```python
from build123d import *

# Parameters (mm, degrees)
BOSS_EXTRUDE1_DEPTH = 126
SKETCH2_R           = 1.5
CUT_EXTRUDE1_DEPTH  = 45
SKETCH3_R           = 1.5
CUT_EXTRUDE3_DEPTH  = 55
CUT_EXTRUDE6_DEPTH  = 45


with BuildPart() as part:
    # Sketch1 → Boss-Extrude1 (new body)
    with BuildSketch(Plane(origin=(0, 0, 0), x_dir=(0, 0, -1), z_dir=(1, 0, 0))):
        Polygon((-95, -3.570472346), (-95, 46.429527654), (-44, 46.429527654), (-44, 51.429527654), (-95, 51.429527654), (-95, 91.429527654), (-25, 91.429527654), (-25, 96.429527654), (-90, 96.429527654), (-100, 96.429527654), (-100, 86.429527654), (-100, -8.570472346), (-90, -8.570472346), (-15, -8.570472346), (-15, -3.570472346), align=None)
    boss_extrude1 = extrude(amount=BOSS_EXTRUDE1_DEPTH)

    # Sketch2 → Cut-Extrude1 (cut)
    with BuildSketch(Plane(origin=(0, 96.429527654, 0), x_dir=(1, 0, 0), z_dir=(0, 1, 0))):
        with Locations(Location((3, -28, 0), (0, 0, 270))):
            Circle(SKETCH2_R)
        with Locations(Location((123, -28, 0), (0, 0, 270))):
            Circle(SKETCH2_R)
    cut_extrude1 = extrude(amount=-CUT_EXTRUDE1_DEPTH, mode=Mode.SUBTRACT)

    # Sketch3 → Cut-Extrude3 (cut)
    with BuildSketch(Plane(origin=(0, 51.429527654, 0), x_dir=(1, 0, 0), z_dir=(0, 1, 0))):
        with Locations(Location((3, -47, 0), (0, 0, 270))):
            Circle(SKETCH3_R)
        with Locations(Location((123, -47, 0), (0, 0, 270))):
            Circle(SKETCH3_R)
        with BuildLine():
            Line((6, -74), (6, -44))
            Line((6, -44), (120, -44))
            Line((120, -44), (120, -74))
            ThreePointArc((120, -74), (117.071067812, -81.071067812), (110, -84))
            Line((110, -84), (16, -84))
            ThreePointArc((16, -84), (8.928932188, -81.071067812), (6, -74))
        make_face()
    cut_extrude3 = extrude(amount=-CUT_EXTRUDE3_DEPTH, mode=Mode.SUBTRACT)

    # Mirror2: Boss-Extrude1, Cut-Extrude1, Cut-Extrude3 across plane
    add(boss_extrude1.mirror(Plane(origin=(0, 0, 15), x_dir=(1, 0, 0), z_dir=(0, 0, -1))))
    add(cut_extrude1.mirror(Plane(origin=(0, 0, 15), x_dir=(1, 0, 0), z_dir=(0, 0, -1))), mode=Mode.SUBTRACT)
    add(cut_extrude3.mirror(Plane(origin=(0, 0, 15), x_dir=(1, 0, 0), z_dir=(0, 0, -1))), mode=Mode.SUBTRACT)

    # Sketch4 → Cut-Extrude6 (cut)
    with BuildSketch(Plane(origin=(0, 96.429527654, 0), x_dir=(1, 0, 0), z_dir=(0, 1, 0))):
        with BuildLine():
            Line((9, -25), (9, -80))
            ThreePointArc((9, -80), (11.928932188, -87.071067812), (19, -90))
            Line((19, -90), (107, -90))
            ThreePointArc((107, -90), (114.071067812, -87.071067812), (117, -80))
            Line((117, -80), (117, -25))
            Line((117, -25), (9, -25))
        make_face()
    cut_extrude6 = extrude(amount=-CUT_EXTRUDE6_DEPTH, mode=Mode.SUBTRACT)

    # Mirror5: Cut-Extrude6 across plane
    add(cut_extrude6.mirror(Plane(origin=(0, 0, 15), x_dir=(1, 0, 0), z_dir=(0, 0, -1))), mode=Mode.SUBTRACT)


solid = part.part
```
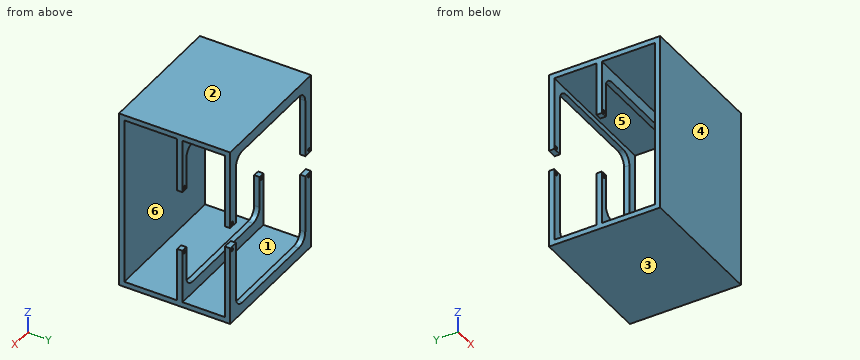
Design review of the part built by this model. Coordinates are the model's own, in mm. Face numbers are marked on the shaded views. A direction names the side the tool comes from. Give positions to 0.01 mm unless a question says otherwise; leave off trailing zeros. Order: outer loops, then holes, each group sorted by start corner. A loop starts at its lowest first (then second) coordinate and runs counter-clockwise, first axis right, second up. Notation, with made-up numbers: (75, 52) -> (84, 52) arc R21 cw to (84, 86) -> close; hole circle Ø2 at (10, 3). An arc over 180 degrees is marked (long way). Write item = value, one per line. Start each with the question number.
(1) We need section C-C on z = -8.5. Write out the cut boundary in (x, y).
(2) Mouldability with a two-part tool opening along Z and no side actions: class the marked faces 3, 4, 5 and 6 as +Z half, -Z half, draft (parallel to the pull), parting line (faces both ways), or undercut.
(3) We need section A-A on z = 60.5. Write out the cut boundary in (x, y).
(4) For pin 1 (3 mm diameter, centred on x = 72, z = -0.5, fed in from +Y), flat-tipped, find the tip position at first contact; note if it passes through.
(5) We need section B-B on y = 34.5. Write out the cut boundary in (x, z).
(6) We need section D-D on x = 42.5. Write out the cut boundary in (y, z), plus the area to 3 significant figures.
(7) For the marked faces 1 and 2, list the 3-axis set-ups (+Z, -Z, +X, -X, +Y, -Y) from which the entire face can be reached by the end or side of a thin tool; tool diameter is ignored.
(8) To check wall thickness, follow line 1 along X through (y, z) = (94.9, 2); line 2 along X through (y, z) = (48, 47); line 3 along Z through (x, y) = (123, 49.1). State the ranges of each line that lie inside material, in increasing order.
Numbers:
q1.outline = (0, -8.57) -> (126, -8.57) -> (126, -3.57) -> (0, -3.57) -> close; (0, 91.43) -> (9, 91.43) -> (9, 96.43) -> (0, 96.43) -> close; (117, 91.43) -> (126, 91.43) -> (126, 96.43) -> (117, 96.43) -> close
q2.face_3 = -Z half
q2.face_4 = draft
q2.face_5 = undercut
q2.face_6 = undercut
q3.outline = (0, -8.57) -> (126, -8.57) -> (126, -3.57) -> (0, -3.57) -> close; (0, 46.43) -> (6, 46.43) -> (6, 51.43) -> (0, 51.43) -> close; (0, 91.43) -> (9, 91.43) -> (9, 96.43) -> (0, 96.43) -> close; (117, 91.43) -> (126, 91.43) -> (126, 96.43) -> (117, 96.43) -> close; (120, 46.43) -> (126, 46.43) -> (126, 51.43) -> (120, 51.43) -> close
q4.pin_1 = -3.57
q5.outline = (0, -70) -> (126, -70) -> (126, -65) -> (0, -65) -> close; (0, 95) -> (126, 95) -> (126, 100) -> (0, 100) -> close
q6.outline = (-8.57, -70) -> (96.43, -70) -> (96.43, -60) -> (91.43, -60) -> (91.43, -65) -> (51.43, -65) -> (51.43, -54) -> (46.43, -54) -> (46.43, -65) -> (-3.57, -65) -> (-3.57, 95) -> (46.43, 95) -> (46.43, 84) -> (51.43, 84) -> (51.43, 95) -> (91.43, 95) -> (91.43, 90) -> (96.43, 90) -> (96.43, 100) -> (-8.57, 100) -> close
q6.area = 2,010 mm^2
q7.face_1 = +X, -X
q7.face_2 = +Z, +X, -X, +Y, -Y
q8.line_1 = 0 to 1.5, 4.5 to 9, 117 to 121.5, 124.5 to 126
q8.line_2 = 0 to 1.5, 4.5 to 6, 120 to 121.5, 124.5 to 126
q8.line_3 = -70 to -18.5, -15.5 to -14, 44 to 45.5, 48.5 to 100
